from build123d import *

# Parameters (mm, degrees)
SKETCH_1_W               = 24
SKETCH_1_H               = 14
SKETCH_1_R               = 1.6
EXTRUDE_1_DEPTH          = 4
SKETCH_3_W               = 24
SKETCH_3_H               = 4
EXTRUDE_2_DEPTH          = 4
SKETCH_5_W               = 24
SKETCH_5_H               = 4
EXTRUDE_3_DEPTH          = 70
SKETCH_8_W               = 24
SKETCH_8_H               = 4
EXTRUDE_4_DEPTH          = 4
SKETCH_9_W               = 24
SKETCH_9_H               = 4
EXTRUDE_5_DEPTH          = 70
EXTRUDE_7_DEPTH          = 4
SKETCH_14_W              = 24
SKETCH_14_H              = 4
CUT_EXTRUDE_2_DEPTH      = 43.2
EXTRUDE_8_DEPTH          = 24
CUT_EXTRUDE_3_DEPTH      = 3
CUT_EXTRUDE_3_DEPTH_BACK = 3
CUT_EXTRUDE_4_DEPTH      = 3
CUT_EXTRUDE_4_DEPTH_BACK = 3
CUT_EXTRUDE_6_REACH      = 90.859
SKETCH_11_R              = 12
SKETCH_11_R_2            = 1.6


with BuildPart() as part:
    # 草图1 → 凸台-拉伸1 (new body)
    with BuildSketch(Plane(origin=(0, 0, 0), x_dir=(1, 0, 0), z_dir=(0, 1, 0))):
        with Locations((12, -7)):
            Rectangle(SKETCH_1_W, SKETCH_1_H)
        with Locations(Location((3, -3, 0), (0, 0, 270))):
            Circle(SKETCH_1_R, mode=Mode.SUBTRACT)
        with Locations(Location((3.000002263, -11, 0), (0, 0, 270))):
            Circle(SKETCH_1_R, mode=Mode.SUBTRACT)
        with Locations(Location((21, -3, 0), (0, 0, 270))):
            Circle(SKETCH_1_R, mode=Mode.SUBTRACT)
        with Locations(Location((21.000002263, -10.308630824, 0), (0, 0, 270))):
            Circle(SKETCH_1_R, mode=Mode.SUBTRACT)
    extrude(amount=EXTRUDE_1_DEPTH)

    # 草图3 → 凸台-拉伸2 (add)
    with BuildSketch(Plane(origin=(0, 0, 0), x_dir=(-1, 0, 0), z_dir=(0, 0, -1))):
        with Locations((-12, 2)):
            Rectangle(SKETCH_3_W, SKETCH_3_H)
    extrude(amount=EXTRUDE_2_DEPTH)

    # 草图5 → 凸台-拉伸3 (add)
    with BuildSketch(Plane(origin=(0, 4, 0), x_dir=(1, 0, 0), z_dir=(0, 1, 0))):
        with Locations((12, 2)):
            Rectangle(SKETCH_5_W, SKETCH_5_H)
    extrude(amount=EXTRUDE_3_DEPTH)

    # 草图8 → 凸台-拉伸4 (add)
    with BuildSketch(Plane.XY.offset(14)):
        with Locations((12, 2)):
            Rectangle(SKETCH_8_W, SKETCH_8_H)
    extrude(amount=EXTRUDE_4_DEPTH)

    # 草图9 → 凸台-拉伸5 (add)
    with BuildSketch(Plane(origin=(0, 4, 0), x_dir=(1, 0, 0), z_dir=(0, 1, 0))):
        with Locations((12, -16)):
            Rectangle(SKETCH_9_W, SKETCH_9_H)
    extrude(amount=EXTRUDE_5_DEPTH)

    # 草图10 → 凸台-拉伸7 (add)
    with BuildSketch(Plane(origin=(0, 0, -4), x_dir=(-1, 0, 0), z_dir=(0, 0, -1))):
        Polygon((-24, 74), (0, 74), (20, 74), (0, 0), (-24, 0), (-44, 74), align=None)
    extrude(amount=-EXTRUDE_7_DEPTH)

    # 草图14 → 切除-拉伸2 (cut)
    with BuildSketch(Plane(origin=(0, 74, 0), x_dir=(1, 0, 0), z_dir=(0, 1, 0))):
        with Locations((12, -16)):
            Rectangle(SKETCH_14_W, SKETCH_14_H)
    extrude(amount=-CUT_EXTRUDE_2_DEPTH, mode=Mode.SUBTRACT)

    # 草图17 → 凸台-拉伸8 (add)
    with BuildSketch(Plane(origin=(24, 0, 0), x_dir=(0, 0, -1), z_dir=(1, 0, 0))):
        Polygon((-14, 30.8), (-14, 14.8), (0, 28.8), (0, 30.8), align=None)
    extrude(amount=-EXTRUDE_8_DEPTH)

    # 草图20 → 切除-拉伸3 (cut, two sides: drawn at the far end of the back side and taken through both)
    with BuildSketch(Plane.ZY.offset(-6).offset(-CUT_EXTRUDE_3_DEPTH_BACK)):
        Polygon((14, 30.8), (14, 14.8), (0, 28.8), (0, 30.8), align=None)
    extrude(amount=CUT_EXTRUDE_3_DEPTH + CUT_EXTRUDE_3_DEPTH_BACK, mode=Mode.SUBTRACT)

    # 草图21 → 切除-拉伸4 (cut, two sides: drawn at the far end of the back side and taken through both)
    with BuildSketch(Plane.ZY.offset(-18).offset(-CUT_EXTRUDE_4_DEPTH_BACK)):
        Polygon((14, 30.8), (14, 14.8), (0, 28.8), (0, 30.8), align=None)
    extrude(amount=CUT_EXTRUDE_4_DEPTH + CUT_EXTRUDE_4_DEPTH_BACK, mode=Mode.SUBTRACT)

    # 草图11 → 切除-拉伸6 (cut, up to next)
    with BuildSketch(Plane(origin=(0, 0, -4), x_dir=(-1, 0, 0), z_dir=(0, 0, -1)), mode=Mode.PRIVATE) as cut_extrude_6_sk1:
        with Locations((-12, 52)):
            Circle(SKETCH_11_R)
    cut_extrude_6_tool1 = extrude(cut_extrude_6_sk1.sketch, amount=-CUT_EXTRUDE_6_REACH, mode=Mode.PRIVATE) & part.part
    # 草图11 → 切除-拉伸6 (cut, up to next)
    with BuildSketch(Plane(origin=(0, 0, -4), x_dir=(-1, 0, 0), z_dir=(0, 0, -1)), mode=Mode.PRIVATE) as cut_extrude_6_sk2:
        with Locations((-27.5, 67.5)):
            Circle(SKETCH_11_R_2)
    cut_extrude_6_tool2 = extrude(cut_extrude_6_sk2.sketch, amount=-CUT_EXTRUDE_6_REACH, mode=Mode.PRIVATE) & part.part
    # 草图11 → 切除-拉伸6 (cut, up to next)
    with BuildSketch(Plane(origin=(0, 0, -4), x_dir=(-1, 0, 0), z_dir=(0, 0, -1)), mode=Mode.PRIVATE) as cut_extrude_6_sk3:
        with Locations((3.5, 67.5)):
            Circle(SKETCH_11_R_2)
    cut_extrude_6_tool3 = extrude(cut_extrude_6_sk3.sketch, amount=-CUT_EXTRUDE_6_REACH, mode=Mode.PRIVATE) & part.part
    # 草图11 → 切除-拉伸6 (cut, up to next)
    with BuildSketch(Plane(origin=(0, 0, -4), x_dir=(-1, 0, 0), z_dir=(0, 0, -1)), mode=Mode.PRIVATE) as cut_extrude_6_sk4:
        with Locations((3.5, 36.5)):
            Circle(SKETCH_11_R_2)
    cut_extrude_6_tool4 = extrude(cut_extrude_6_sk4.sketch, amount=-CUT_EXTRUDE_6_REACH, mode=Mode.PRIVATE) & part.part
    # 草图11 → 切除-拉伸6 (cut, up to next)
    with BuildSketch(Plane(origin=(0, 0, -4), x_dir=(-1, 0, 0), z_dir=(0, 0, -1)), mode=Mode.PRIVATE) as cut_extrude_6_sk5:
        with Locations((-27.5, 36.5)):
            Circle(SKETCH_11_R_2)
    cut_extrude_6_tool5 = extrude(cut_extrude_6_sk5.sketch, amount=-CUT_EXTRUDE_6_REACH, mode=Mode.PRIVATE) & part.part
    add(cut_extrude_6_tool1.solids().sort_by_distance((12, 52, -4))[0], mode=Mode.SUBTRACT)
    add(cut_extrude_6_tool2.solids().sort_by_distance((27.5, 67.5, -4))[0], mode=Mode.SUBTRACT)
    add(cut_extrude_6_tool3.solids().sort_by_distance((-3.5, 67.5, -4))[0], mode=Mode.SUBTRACT)
    add(cut_extrude_6_tool4.solids().sort_by_distance((-3.5, 36.5, -4))[0], mode=Mode.SUBTRACT)
    add(cut_extrude_6_tool5.solids().sort_by_distance((27.5, 36.5, -4))[0], mode=Mode.SUBTRACT)


solid = part.part
Work out the finished part from the listing and answer in its coordinate system (mm). A direction names the side the tool comes from. Round coordinates to 2 decimals unless told otherwise and drop trailing zeros. Loops run counter-clockwise (first coordinate to the right, second up) from the corner with the lowest first, then second, coordinate; pieces in that order, holes last. Notation, with made-up numbers: (-8, -28.75) - (38, -28.75) arc R13 cw to (38, -16.75) - close; hole circle Ø10 at (76.5, 71.25). An arc over 180 degrees is marked (long way). Use one line per item in the form item = value. Start each with the question number.
(1) Determine the mould class of faces 1 (the face through (12, 30.8, 11)), 2 (the face through (3, 25, 9)), 3 (the face through (0, 19, 11)) for opening direction X: +X half, -X half, draft (parallel to the pull), parting line (faces both ways), or undercut.
(2) Flat-ended cylindrical pins translate along their axes: P1, Ø11, axis at y = 25, z = 6.5, coming from the -X side; P2, Ø5, axis at x = 27.5, y = 36.5, coming from the -Z side; P3, Ø9, axis at x = 7.5, z = 10.5, coming from the +Y side; P4, Ø10, axis at y = 66, z = 2.5, coming from the +X side. Find the tip coordinate at first contact, or state that the pin passes through.
(3) Consider line 1 (X direction, y = 1.4, z = 3); line 2 (X direction, y = 67.5, z = -2.1); line 3 (Z direction, x = 1.5, y = 38). Determine where each line is inside the solid, lowest interval first.
(4) Find section A-A on z = 7.5. Determine the outline of the cut face in (x, y), and give its area (3 significant figures).
(5) Find section B-B on x = 12. Determine the outline of the cut face in (y, z), and give its area (3 significant figures).
(6) Find section D-D on x = 27.5. Determine the outline of the cut face in (y, z).
(7) Which of the six approach directions +Z, -Z, +X, -X, +Y, -Y give full straight-line access (tool end or side, diameter ignored) to faces 4 (the face through (-3.292, 69.086, -2.028)), 5 (the face through (24, 19, 11)), 6 (the face through (12, 4, 7)), 7 (the face through (3.07, 1.97, 9.4))?
(8) Find section C-C on y = 67.5. Determine the outline of the cut face in (x, z).
Answer list:
q1.face_1 = draft
q1.face_2 = undercut
q1.face_3 = -X half
q2.P1 = 0
q2.P2 = -4
q2.P3 = 30.8
q2.P4 = 43.01
q3.line_1 = 0 to 1.4, 4.6 to 19.4, 22.6 to 24
q3.line_2 = -18.24 to -5.1, -1.9 to 25.9, 29.1 to 42.24
q3.line_3 = -4 to 0
q4.outline = (0, 0) - (24, 0) - (24, 4) - (0, 4) - close; (0, 21.3) - (3, 21.3) - (3, 30.8) - (0, 30.8) - close; (9, 21.3) - (15, 21.3) - (15, 30.8) - (9, 30.8) - close; (21, 21.3) - (24, 21.3) - (24, 30.8) - (21, 30.8) - close
q4.area = 210 mm^2
q5.outline = (0, -4) - (40, -4) - (40, 0) - (30.8, 0) - (30.8, 18) - (0, 18) - close; (64, -4) - (74, -4) - (74, 0) - (64, 0) - close; hole (4, 0) - (28.8, 0) - (14.8, 14) - (4, 14) - close
q5.area = 505 mm^2
q6.outline = (12.95, -4) - (34.9, -4) - (34.9, 0) - (12.95, 0) - close; (38.1, -4) - (65.9, -4) - (65.9, 0) - (38.1, 0) - close; (69.1, -4) - (74, -4) - (74, 0) - (69.1, 0) - close
q7.face_4 = +Z, -Z
q7.face_5 = +Z, +X, +Y, -Y
q7.face_6 = +X, -X
q7.face_7 = -Y
q8.outline = (-18.24, -4) - (-5.1, -4) - (-5.1, 0) - (-18.24, 0) - close; (-1.9, -4) - (25.9, -4) - (25.9, 0) - (-1.9, 0) - close; (29.1, -4) - (42.24, -4) - (42.24, 0) - (29.1, 0) - close
